The listing builds one solid part. Answer for the finished solid, in the listing's coordinates (mm). Face numbers are marked on the shaded views. A direction names the side the tool comes from. Coordinates: 2 decimals unless noted, no trailing zeros. Write each loop counter-clockwise with the first axis right and the second up, starting at its lowest first coordinate (ties: lowest second). Pieces come first, ordered by that corner, then holes. Notation, with made-up numbers: M 37,18 L 71,18 A23 cw 71,29 Z; hole C 17,3 d6. An arc over 180 degrees is marked long. Answer as CSV lines item,"result". Start each with the question number.
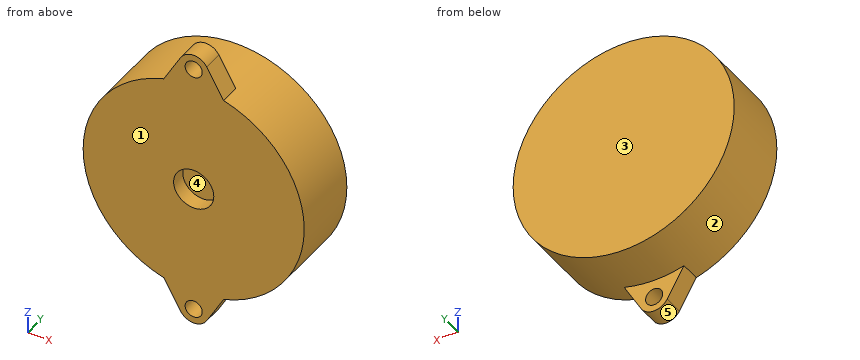
Autodesk Inventor part; units mm, degrees
ref_plane "YZ Plane" through (0, 0, 0) normal (1, 0, 0) x (0, 1, 0)
ref_plane "XZ Plane" through (0, 0, 0) normal (0, 1, 0) x (-1, 0, 0)
ref_plane "XY Plane" through (0, 0, 0) normal (0, 0, 1) x (1, 0, 0)
sketch "Sketch1" plane through (0, 0, 0) normal (0, 1, 0) x (-1, 0, 0)
  circle A0 centre (0, 0) radius 22
  circle A1 centre (0, -25.5) radius 3
  line L0 (2.5981, -27) -> (5.9598, -21.1774)
  line L1 (-2.5981, -27) -> (-5.9598, -21.1774)
  line L2 (30.8, 0) -> (-30.8, 0)
  circle A2 centre (0, 25.5) radius 3
  line L3 (2.5981, 27) -> (5.9598, 21.1774)
  line L4 (-2.5981, 27) -> (-5.9598, 21.1774)
  point P0 (5.9598, 21.1774)
  point P1 (-5.9598, 21.1774)
  dimension "d0" = 44
  dimension "d1" = 60
  dimension "d2" = 6
  dimension "d3" = 51
extrude "Extrusion1" add sketch "Sketch1" along normal blind 14 contours L2 A0 | A0 L2
extrude "Extrusion2" add sketch "Sketch1" along normal blind 4 contours A0 L4 A2 L3 | L0 A1 L1 A0 | A2 | A1
hole "Hole1" at (0, 0, -25.5) at (0, 0, 25.5) direction (0, 1, 0) diameter 3.4 depth 4
sketch "Sketch2" plane through (0, 0, 0) normal (0, 1, 0) x (1, 0, 0)
  circle A0 centre (0, 0) radius 4
  dimension "d15" = 8
extrude "Extrusion3" cut sketch "Sketch2" along normal blind 3
properties part number "speaker"
1) For a pull along X with two mould halves and no side action, classify the marked faces 3, 4 and 5 as +X half, -X half, draft (parallel to the pull), parting line (faces both ways), or undercut.
2) The part is cut by section B-B (z = 25.5). Determine the outline of the cut face in (x, y).
3) The part is cut by section C-C (y = 2). Determine the outline of the cut face in (x, z).
4) The part is cut by section D-D (z = 0). Determine the outline of the cut face in (x, y).
5) The part is cut by section A-A (x = 0). Determine the outline of the cut face in (y, z).
6) Find the intervals of material crossed by line 1 (X direction, y = 1.35, z = 0); line 2 (X direction, y = 2.7, z = 25.5); line 3 (Z direction, x = 6, y = 4.25), in increasing order. Write a range as from..to.
7) Which of the six approach directions +Z, -Z, +X, -X, +Y, -Y give full straight-line access (tool end or side, diameter ignored) to the marked faces 1 and 2?
8) Each of these flat-tipped pins is pushed along its axis until it touches: P1, Ø1.5, axis at y = 6, z = 10, coming from the -X side; P2, Ø5, axis at x = 7.5, y = 3.5, coming from the -Z side; P3, Ø5, axis at y = 7, z = 15.5, coming from the +X side; P4, Ø3, axis at x = 0, z = -25.5, coming from the -Y side. Where does it stop, or does it pass through?
Completed:
1,face 3,"draft"
1,face 4,"undercut"
1,face 5,"parting line"
2,outline,"M -3.46,0 L -1.7,0 L -1.7,4 L -3.46,4 Z; M 1.7,0 L 3.46,0 L 3.46,4 L 1.7,4 Z"
3,outline,"M -5.96,-21.18 L -2.6,-27 A3 ccw 2.6,-27 L 5.96,-21.18 A22 ccw 5.96,21.18 L 2.6,27 A3 ccw -2.6,27 L -5.96,21.18 A22 ccw Z; hole C 0,0 d8; hole C 0,-25.5 d3.4; hole C 0,25.5 d3.4"
4,outline,"M -22,0 L -4,0 L -4,3 L 4,3 L 4,0 L 22,0 L 22,14 L -22,14 Z"
5,outline,"M 0,-28.5 L 4,-28.5 L 4,-27.2 L 0,-27.2 Z; M 0,-23.8 L 4,-23.8 L 4,-22 L 14,-22 L 14,22 L 4,22 L 4,23.8 L 0,23.8 L 0,4 L 3,4 L 3,-4 L 0,-4 Z; M 0,27.2 L 4,27.2 L 4,28.5 L 0,28.5 Z"
6,line 1,"-22..-4, 4..22"
6,line 2,"-3.46..-1.7, 1.7..3.46"
6,line 3,"-21.17..21.17"
7,face 1,"+Z, -Z, +X, -X, -Y"
7,face 2,"+Y"
8,P1,"x = -19.96"
8,P2,"z = -22.84"
8,P3,"x = 17.75"
8,P4,"through"
